from build123d import *

# Parameters (mm, degrees)
F0_W     = 101.6
F0_H     = 40.64
F1_DEPTH = 9.525
F2_R     = 1.27
F3_DEPTH = 40.641


with BuildPart() as f1:
    # F0 (on Front) → F1 (new body)
    with BuildSketch(Plane.XZ):
        Rectangle(F0_W, F0_H)
    extrude(amount=-F1_DEPTH)

    # F2 (on face) → F3 (cut, through all)
    with BuildSketch(Plane(origin=(0, 0, -20.32), x_dir=(1, 0, 0), z_dir=(0, 0, -1))):
        with Locations((-40.20207, -4.601012)):
            Circle(F2_R)
        with Locations((0, -4.601012)):
            Circle(F2_R)
        with Locations((39.93931, -4.601012)):
            Circle(F2_R)
    extrude(amount=-F3_DEPTH, mode=Mode.SUBTRACT)


solid = f1.part
The listing builds one solid part. Answer for the finished solid, in the listing's coordinates (mm). Round coordinates to 2 decimals unless told otherwise and drop trailing zeros. Order: outer loops, then holes, each group sorted by start corner. A loop starts at its lowest first (then second) coordinate and runs counter-clockwise, first axis right, second up. Notation, with made-up numbers: (88, 55.5) -> (123, 55.5) arc R11 cw to (123, 75.5) -> close; hole circle Ø1 at (27, 88.25). An arc over 180 degrees is marked (long way). One line per item, written item: value.
Item 1: Straight lines are drawn through the part: L1, parallel to X at y = 4.75, z = 18; L2, parallel to Y at x = 0, z = 7.5 (3 decimals); L3, parallel to X at y = 3.75, z = 8. For each, find the intervals that lie inside material, in ascending order.
Taken from the geometry:
L1: x = -50.8 to -41.46, -38.94 to -1.26, 1.26 to 38.68, 41.2 to 50.8
L2: y = 0 to 3.331, 5.871 to 9.525
L3: x = -50.8 to -41.14, -39.26 to -0.94, 0.94 to 39, 40.88 to 50.8
Item 2: Find section B-B, the plane z = 4.5. Give the vertices of the cut face in (x, y) (3 decimals), then the cut area to 3 significant figures.
Taken from the geometry:
outline: (-50.8, 0) -> (50.8, 0) -> (50.8, 9.525) -> (-50.8, 9.525) -> close; hole circle Ø2.54 at (-40.202, 4.601); hole circle Ø2.54 at (0, 4.601); hole circle Ø2.54 at (39.939, 4.601)
area: 953 mm2
Item 3: Given P1, Ø4, axis at x = 0, y = 4.6, coming from the +Z side, flat-ended and moving along its own axis, determine where the tip first touches the part or whether it passes through.
Taken from the geometry:
P1: stops at z = 20.32
Item 4: Find section A-A, the plane x = 0. Give the vertices of the cut face in (y, z) (3 decimals), then the cut area to 3 significant figures.
Taken from the geometry:
outline: (0, -20.32) -> (3.331, -20.32) -> (3.331, 20.32) -> (0, 20.32) -> close; (5.871, -20.32) -> (9.525, -20.32) -> (9.525, 20.32) -> (5.871, 20.32) -> close
area: 284 mm2
Item 5: For a pull along Y with two mould halves and no side action, classify faces 1 (the flat face through (-1, 6, 20.32)), 2 (the cylindrical face through (41.11, 5.09, -0.28)), 3 (the cylindrical face through (-0.28, 5.84, -0.28)), 4 (the flat face through (-1, 0, 0)) as released by +Y, released by -Y, zero draft, split by the parting line, or undercut.
Taken from the geometry:
face 1: zero draft
face 2: undercut
face 3: undercut
face 4: released by -Y
